For this review, take the finished solid that the model builds, in its own axes (mm). A direction names the side the tool comes from. Give positions to 0.01 mm unless a question says otherwise; leave off trailing zeros. Order: outer loops, then holes, each group sorted by start corner. A loop starts at its lowest first (then second) coordinate and runs counter-clockwise, first axis right, second up.
from build123d import *

# Parameters (mm, degrees)
F0_R     = 12.7
F1_DEPTH = 25.4
F2_R     = 12.7
F3_DEPTH = 50.8


with BuildPart() as f1:
    # F0 (on Top) → F1 (new body)
    with BuildSketch(Plane.XY):
        with BuildLine():
            Line((-33.125833, -5.772527), (-7.9375, -17.31758))
            ThreePointArc((-7.9375, -17.31758), (0, -19.05), (7.9375, -17.31758))
            Line((7.9375, -17.31758), (33.125833, -5.772527))
            ThreePointArc((33.125833, -5.772527), (36.83, 0), (33.125833, 5.772527))
            Line((33.125833, 5.772527), (7.9375, 17.31758))
            ThreePointArc((7.9375, 17.31758), (0, 19.05), (-7.9375, 17.31758))
            Line((-7.9375, 17.31758), (-33.125833, 5.772527))
            ThreePointArc((-33.125833, 5.772527), (-36.83, 0), (-33.125833, -5.772527))
        make_face()
        Circle(F0_R, mode=Mode.SUBTRACT)
    extrude(amount=F1_DEPTH)

    # F2 (on face) → F3 (join)
    with BuildSketch(Plane.XY.offset(25.4)):
        with BuildLine():
            Line((13.97, -12.95151), (13.97, 12.95151))
            ThreePointArc((13.97, 12.95151), (11.169167, 15.432181), (7.9375, 17.31758))
            ThreePointArc((7.9375, 17.31758), (0, 19.05), (-7.9375, 17.31758))
            ThreePointArc((-7.9375, 17.31758), (-11.169167, 15.432181), (-13.97, 12.95151))
            Line((-13.97, 12.95151), (-13.97, -12.95151))
            ThreePointArc((-13.97, -12.95151), (-11.169167, -15.432181), (-7.9375, -17.31758))
            ThreePointArc((-7.9375, -17.31758), (0, -19.05), (7.9375, -17.31758))
            ThreePointArc((7.9375, -17.31758), (11.169167, -15.432181), (13.97, -12.95151))
        make_face()
        Circle(F2_R, mode=Mode.SUBTRACT)
    extrude(amount=F3_DEPTH)


solid = f1.part
1) We need section B-B on y = 0. Give the boundary of the cut face in (x, z).
Answer sheet:
outline: (-36.83, 0) - (-12.7, 0) - (-12.7, 76.2) - (-13.97, 76.2) - (-13.97, 25.4) - (-36.83, 25.4) - close; (12.7, 0) - (36.83, 0) - (36.83, 25.4) - (13.97, 25.4) - (13.97, 76.2) - (12.7, 76.2) - close
2) Tool access review of faces 1 (the face through (-1, 13, 0)), 2 (the face through (13.97, 0, 50)), 3 (the face through (-13.97, 0, 50)): name each direction out of +Z, -Z, +X, -X, +Y, -Y from which nothing blocks a thin tool from reaching the whole face with its end or side.
Answer sheet:
face 1: -Z, +X, -X, +Y, -Y
face 2: +Z, +X, +Y, -Y
face 3: +Z, -X, +Y, -Y
3) To check wall thickness, follow line 1 (Y direction, x = 0, z = 54); line 2 (Z direction, x = 33, y = 1); line 3 (Y direction, x = 4, z = 62). State the ranges of each line that lie inside material, in increasing order.
Answer sheet:
line 1: y = -19.05 to -12.7, 12.7 to 19.05
line 2: z = 0 to 25.4
line 3: y = -18.63 to -12.05, 12.05 to 18.63
4) We need section D-D on z = 20.5. Give the boundary of the cut face in (x, y), then the cut area to 3 significant figures.
Answer sheet:
outline: (-33.13, -5.77) - (-7.94, -17.32) arc R19.05 ccw to (7.94, -17.32) - (33.13, -5.77) arc R6.35 ccw to (33.13, 5.77) - (7.94, 17.32) arc R19.05 ccw to (-7.94, 17.32) - (-33.13, 5.77) arc R6.35 ccw to start; hole circle Ø25.4 at (0, 0)
area: 1,300 mm2
5) We need section C-C on x = 0. Give the boundary of the cut face in (y, z), then the cut area to 3 significant figures.
Answer sheet:
outline: (-19.05, 0) - (-12.7, 0) - (-12.7, 76.2) - (-19.05, 76.2) - close; (12.7, 0) - (19.05, 0) - (19.05, 76.2) - (12.7, 76.2) - close
area: 968 mm2
6) We need section A-A on z = 48.5. Give the boundary of the cut face in (x, y).
Answer sheet:
outline: (-13.97, -12.95) arc R19.05 ccw to (-7.94, -17.32) arc R19.05 ccw to (7.94, -17.32) arc R19.05 ccw to (13.97, -12.95) - (13.97, 12.95) arc R19.05 ccw to (7.94, 17.32) arc R19.05 ccw to (-7.94, 17.32) arc R19.05 ccw to (-13.97, 12.95) - close; hole circle Ø25.4 at (0, 0)
7) Clearance check with flat-ended pins moving along their axes: pin 1 (12 mm diameter, centred on y = -9, z = 45, fed in from -X); pin 2 (12 mm diameter, centred on x = 23, z = 56.5, fed in from -Y); pin 3 (8 mm diameter, centred on y = -5, z = 15, fed in from -X); pin 4 (3 mm diameter, centred on x = -23, y = -8.5, fed in from +Z). State where each tip first meets the part, or that it passes through.
Answer sheet:
pin 1: stops at x = -13.97
pin 2: passes through
pin 3: stops at x = -36.75
pin 4: stops at z = 25.4
